Part print with two shaded views. Sizes in mm from the minimum x, y, z corner. Give positions to 0.01 mm unless a question says otherwise; leave off trailing zeros. Write each loop counter-clockwise with the first axis right and the second up, starting at its lowest first coordinate (ties: lowest second). Pieces come first, ordered by that corner, then holes.
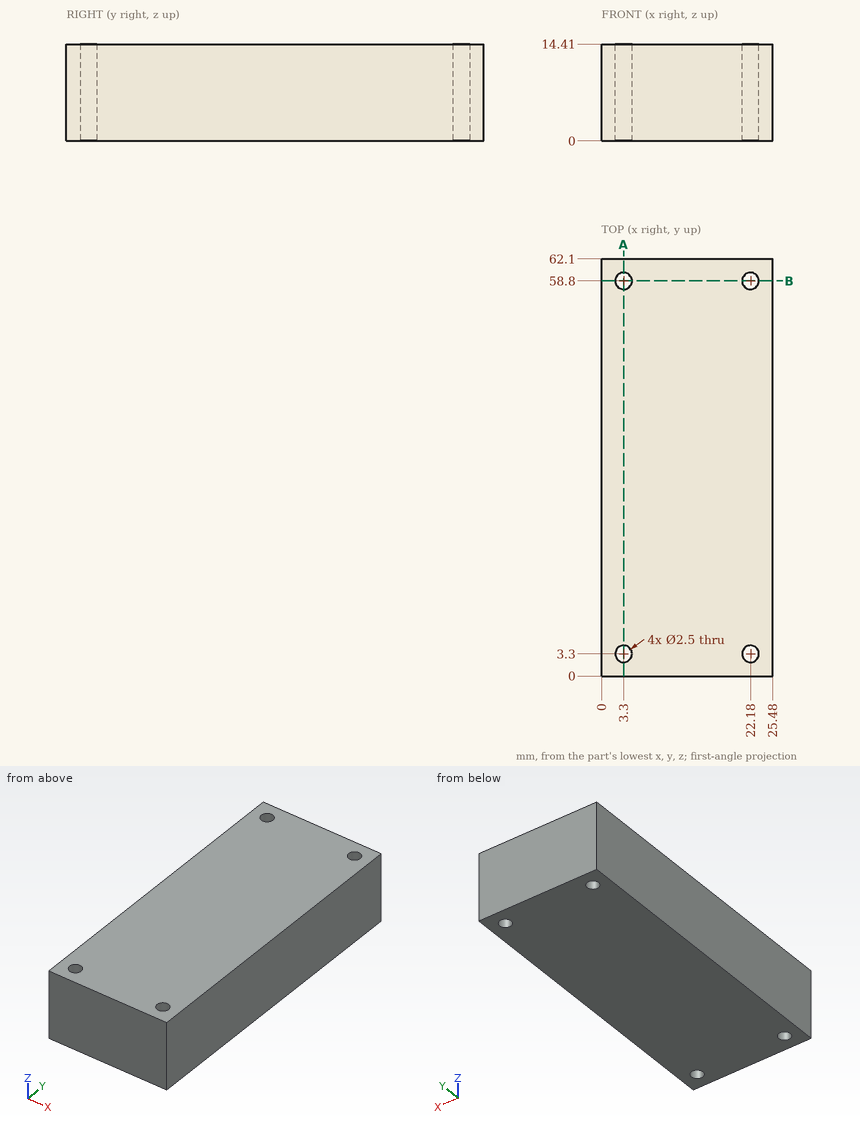
1) Pin check, flat tip, straight feed: pin 1 Ø2 at (x, y) = (22.18, 3.3) entering from +Z. Stop position of the tip, or through.
Answers follow:
pin 1: passes through
2) Wall check: L1, parallel to Y at x = 4, z = 4.5. Give the ranges that are in metal, low to high.
Answers follow:
L1: y = 0 to 2.26, 4.34 to 57.76, 59.84 to 62.1
3) Saw through at B-B, the plane y = 58.8. Write the cut outline in (x, z), then the cut area to 3 significant figures.
Answers follow:
outline: (0, 0) - (2.05, 0) - (2.05, 14.41) - (0, 14.41) - close; (4.55, 0) - (20.93, 0) - (20.93, 14.41) - (4.55, 14.41) - close; (23.43, 0) - (25.48, 0) - (25.48, 14.41) - (23.43, 14.41) - close
area: 295 mm2
4) Saw through at A-A, the plane x = 3.3. Write the cut outline in (y, z), then the cut area to 3 significant figures.
Answers follow:
outline: (0, 0) - (2.05, 0) - (2.05, 14.41) - (0, 14.41) - close; (4.55, 0) - (57.55, 0) - (57.55, 14.41) - (4.55, 14.41) - close; (60.05, 0) - (62.1, 0) - (62.1, 14.41) - (60.05, 14.41) - close
area: 823 mm2
